Geometry check sheet. Reference: the model listing, model coordinates, mm. Round coordinates to 2 decimals unless told otherwise and drop trailing zeros. Loops run counter-clockwise (first coordinate to the right, second up) from the corner with the lowest first, then second, coordinate; pieces in that order, holes last. Notation, with made-up numbers: (84.5, 60.25) -> (88.5, 60.25) arc R36 cw to (88.5, 97.25) -> close; hole circle Ø10 at (-1, 83). An arc over 180 degrees is marked (long way). Use a Markdown table: item, result. Add a question column.
Q1. Sectioned sample at B-B, the plane z = 12.5. Give the number of separate pieces and of enclosed holes in the cut face, then the cut area to 3 significant figures.
Q2. Sectioned sample at A-A, the plane x = -51.5. Enter the section's corners in (y, z).
Q3. Material ranges on L1, parallel to Y at x = -37.5, z = 5.75; L2, parallel to Y at x = -48.5, z = 13.5; L3, parallel to X at y = 102, z = 10, recorded low to high.
Q4. Gauge pin test, flat ends, axial feed: P1, Ø4, axis at x = -121.98, y = 134.3, coming from the +Z side; P2, Ø4, axis at x = -73, y = 70, coming from the +Z side; P3, Ø3.5, axis at x = -98.5, y = 133.5, coming from the +Z side. Record the tip position at first contact, or that the pin passes through.
```python
from build123d import *

# Parameters (mm, degrees)
F0_W           = 250
F0_H           = 230
F1_DEPTH       = 15
F3_D           = 6.6
F3_CBORE_D     = 11.25
F3_CBORE_DEPTH = 6
F4_DEPTH       = 5
F5_D           = 6.6
F6_DEPTH       = 5


with BuildPart() as f1:
    # F0 (on Top) → F1 (new body)
    with BuildSketch(Plane.XY):
        with Locations((-61.9829781353, 69.301483577)):
            Rectangle(F0_W, F0_H)
    extrude(amount=F1_DEPTH)

    # F3 (through all)
    with Locations(Plane.XY.offset(15)):
        with Locations((-121.9829781353, 134.301483577), (-96.9829781353, 134.301483577), (-86.9829781353, 124.301483577), (-86.9829781353, 99.301483577), (-36.9829781353, 99.301483577), (-36.9829781353, 124.301483577), (-26.9829781353, 134.301483577), (-1.9829781353, 134.301483577)):
            CounterBoreHole(F3_D / 2, F3_CBORE_D / 2, F3_CBORE_DEPTH)

    # F2 (on face) → F4 (cut)
    with BuildSketch(Plane.XY.offset(15)):
        with BuildLine():
            Line((-40.9829781353, 72.301483577), (-61.9829781353, 72.301483577))
            Line((-61.9829781353, 72.301483577), (-61.9829781353, 64.301483577))
            Line((-61.9829781353, 64.301483577), (-40.9829781353, 64.301483577))
            ThreePointArc((-40.9829781353, 64.301483577), (-38.1545510106, 65.4730564522), (-36.9829781353, 68.301483577))
            ThreePointArc((-36.9829781353, 68.301483577), (-38.1545510106, 71.1299107017), (-40.9829781353, 72.301483577))
        make_face()
        with BuildLine():
            Line((-61.9829781353, 64.301483577), (-61.9829781353, 72.301483577))
            Line((-61.9829781353, 72.301483577), (-82.9829781353, 72.301483577))
            ThreePointArc((-82.9829781353, 72.301483577), (-85.8114052601, 71.1299107017), (-86.9829781353, 68.301483577))
            ThreePointArc((-86.9829781353, 68.301483577), (-85.8114052601, 65.4730564522), (-82.9829781353, 64.301483577))
            Line((-82.9829781353, 64.301483577), (-61.9829781353, 64.301483577))
        make_face()
    extrude(amount=-F4_DEPTH, mode=Mode.SUBTRACT)

    # F5 (through all)
    with Locations(Plane.XY.offset(15)):
        with Locations((53.0170218647, 43.301483577), (-1.9829781353, 43.301483577), (53.0170218647, 94.301483577), (-36.9829781353, -21.698516423), (-86.9829781353, -21.698516423), (-121.9829781353, 43.301483577), (-176.9829781353, 43.301483577), (-176.9829781353, 94.301483577)):
            Hole(F5_D / 2)

    # F2 (on face) → F6 (cut)
    with BuildSketch(Plane.XY.offset(15)):
        with BuildLine():
            Line((-61.9829781353, 155.301483577), (-61.9829781353, 163.301483577))
            Line((-61.9829781353, 163.301483577), (-82.9829781353, 163.301483577))
            ThreePointArc((-82.9829781353, 163.301483577), (-85.8114052601, 162.1299107017), (-86.9829781353, 159.301483577))
            ThreePointArc((-86.9829781353, 159.301483577), (-85.8114052601, 156.4730564522), (-82.9829781353, 155.301483577))
            Line((-82.9829781353, 155.301483577), (-61.9829781353, 155.301483577))
        make_face()
        with BuildLine():
            Line((-40.9829781353, 163.301483577), (-61.9829781353, 163.301483577))
            Line((-61.9829781353, 163.301483577), (-61.9829781353, 155.301483577))
            Line((-61.9829781353, 155.301483577), (-40.9829781353, 155.301483577))
            ThreePointArc((-40.9829781353, 155.301483577), (-38.1545510106, 156.4730564522), (-36.9829781353, 159.301483577))
            ThreePointArc((-36.9829781353, 159.301483577), (-38.1545510106, 162.1299107017), (-40.9829781353, 163.301483577))
        make_face()
    extrude(amount=-F6_DEPTH, mode=Mode.SUBTRACT)


solid = f1.part
```
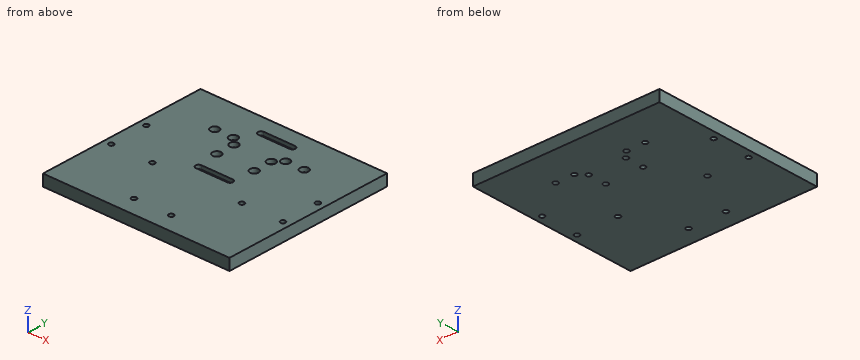
Values:
| question | item | result |
|---|---|---|
| 1 | separate pieces | 1 |
| 1 | enclosed holes | 18 |
| 1 | area | 55,700 mm^2 |
| 2 | outline | (-45.7, 0) -> (184.3, 0) -> (184.3, 15) -> (163.3, 15) -> (163.3, 10) -> (155.3, 10) -> (155.3, 15) -> (72.3, 15) -> (72.3, 10) -> (64.3, 10) -> (64.3, 15) -> (-45.7, 15) -> close |
| 3 | L1 | -45.7 to -24.96, -18.44 to 96.04, 102.56 to 121.04, 127.56 to 184.3 |
| 3 | L2 | -45.7 to 64.3, 72.3 to 155.3, 163.3 to 184.3 |
| 3 | L3 | -186.98 to -91.92, -82.05 to -41.92, -32.05 to 63.02 |
| 4 | P1 | through |
| 4 | P2 | z = 10 |
| 4 | P3 | z = 9 |
